Model file for the job. Use its own axes, mm. Face numbers are marked on the shaded views. A direction names the side the tool comes from. Round coordinates to 2 decimals unless told otherwise and drop trailing zeros. Loops run counter-clockwise (first coordinate to the right, second up) from the corner with the lowest first, then second, coordinate; pieces in that order, holes last. Notation, with made-up numbers: M 79.25,59.5 L 126.25,59.5 A29 ccw 126.25,96.5 Z; hole C 79.5,57.5 d1. An arc over 180 degrees is marked long. Answer in a Markdown table with one row per item.
from build123d import *

# Parameters (mm, degrees)
BOSS_EXTRUDE1_DEPTH = 51
CUT_EXTRUDE2_DEPTH  = 51
SKETCH4_R           = 1.625
CUT_EXTRUDE3_DEPTH  = 51
CHAMFER1_SIZE       = 5
FILLET1_R           = 2
SKETCH5_W           = 20.5
SKETCH5_H           = 40.5
CUT_EXTRUDE4_DEPTH  = 10
RIB1_REACH          = 100.443
SKETCH6_WALL_W      = 251.096798658
SKETCH6_WALL_H      = 4
SKETCH7_R           = 1.5
CUT_EXTRUDE5_DEPTH  = 10
SKETCH2_R           = 11.125
CUT_EXTRUDE6_DEPTH  = 10


with BuildPart() as part:
    # Sketch1 → Boss-Extrude1 (new body)
    with BuildSketch(Plane(origin=(0, 0, 0), x_dir=(0, 0, -1), z_dir=(1, 0, 0))):
        Polygon((0, 0), (0, 67), (4, 67), (4, 4), (51, 4), (51, 0), align=None)
    extrude(amount=BOSS_EXTRUDE1_DEPTH)

    # Sketch3 → Cut-Extrude2 (cut)
    with BuildSketch(Plane(origin=(0, 4, 0), x_dir=(1, 0, 0), z_dir=(0, 1, 0))):
        with BuildLine():
            Line((8.34, 40.85), (8.34, 11.15))
            ThreePointArc((8.34, 11.15), (10.49, 9), (12.64, 11.15))
            Line((12.64, 11.15), (12.64, 40.85))
            ThreePointArc((12.64, 40.85), (10.49, 43), (8.34, 40.85))
        make_face()
        with BuildLine():
            Line((38.36, 40.85), (38.36, 11.15))
            ThreePointArc((38.36, 11.15), (40.51, 9), (42.66, 11.15))
            Line((42.66, 11.15), (42.66, 40.85))
            ThreePointArc((42.66, 40.85), (40.51, 43), (38.36, 40.85))
        make_face()
    extrude(amount=-CUT_EXTRUDE2_DEPTH, mode=Mode.SUBTRACT)

    # Sketch4 → Cut-Extrude3 (cut)
    with BuildSketch(Plane.XY):
        with Locations((10, 46.5)):
            Circle(SKETCH4_R)
        with Locations((41, 46.5)):
            Circle(SKETCH4_R)
        with Locations((41, 15.5)):
            Circle(SKETCH4_R)
        with Locations((10, 15.5)):
            Circle(SKETCH4_R)
    extrude(amount=-CUT_EXTRUDE3_DEPTH, mode=Mode.SUBTRACT)

    # Chamfer1
    chamfer1_edges = [part.edges().sort_by_distance(p)[0] for p in [
        (51, 67, -2),
        (0, 67, -2),
        (0, 2, -51),
        (51, 2, -51),
    ]]
    chamfer(chamfer1_edges, length=CHAMFER1_SIZE)

    # Fillet1
    fillet1_edges = [part.edges().sort_by_distance(p)[0] for p in [
        (46, 2, -51),
        (5, 2, -51),
        (0, 62, -2),
        (0, 2, -46),
        (51, 62, -2),
        (51, 2, -46),
        (5, 67, -2),
        (46, 67, -2),
    ]]
    fillet(fillet1_edges, radius=FILLET1_R)

    # Sketch5 → Cut-Extrude4 (cut)
    with BuildSketch(Plane(origin=(0, 0, -4), x_dir=(-1, 0, 0), z_dir=(0, 0, -1))):
        with Locations((-25.5, 36.25)):
            Rectangle(SKETCH5_W, SKETCH5_H)
    extrude(amount=-CUT_EXTRUDE4_DEPTH, mode=Mode.SUBTRACT)

    # Sketch6 wall → Rib1 (add, up to next)
    with BuildSketch(Plane(origin=(51, 21.375514331, -23.483064602), x_dir=(0, -0.665587686923, -0.746319657397), z_dir=(0, 0.746319657397, -0.665587686923)), mode=Mode.PRIVATE) as rib1_sk1:
        with Locations((0, 2)):
            Rectangle(SKETCH6_WALL_W, SKETCH6_WALL_H)
    rib1_tool1 = extrude(rib1_sk1.sketch, amount=-RIB1_REACH, mode=Mode.PRIVATE) - part.part
    rib1 = rib1_tool1.solids().sort_by_distance((51, 21.375514331, -23.483064602))[0]
    add(rib1)

    # Mirror1: Rib1 across plane
    add(rib1.mirror(Plane.ZY.offset(-25.5)))

    # Sketch7 → Cut-Extrude5 (cut)
    with BuildSketch(Plane(origin=(0, 0, -4), x_dir=(-1, 0, 0), z_dir=(0, 0, -1))):
        with Locations(Location((-31.45, 60.8, 0), (0, 0, 90))):
            Circle(SKETCH7_R)
        with Locations(Location((-19.55, 60.8, 0), (0, 0, 90))):
            Circle(SKETCH7_R)
        with Locations(Location((-31.45, 11.7, 0), (0, 0, 90))):
            Circle(SKETCH7_R)
        with Locations(Location((-19.55, 11.7, 0), (0, 0, 90))):
            Circle(SKETCH7_R)
    extrude(amount=-CUT_EXTRUDE5_DEPTH, mode=Mode.SUBTRACT)

    # Sketch2 → Cut-Extrude6 (cut)
    with BuildSketch(Plane.XY):
        with Locations((25.5, 31)):
            Circle(SKETCH2_R)
    extrude(amount=-CUT_EXTRUDE6_DEPTH, mode=Mode.SUBTRACT)


solid = part.part
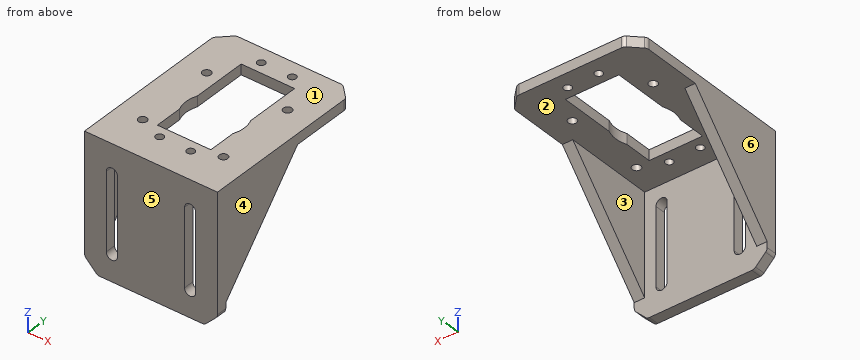
1. Tool access for the marked faces 1 and 2: list every direction of +Z, -Z, +X, -X, +Y, -Y with a clear straight run to the whole face (end or side of a thin tool).
Verdict:
| item | result |
|---|---|
| face 1 | +Z, +X, -X, +Y, -Y |
| face 2 | -Z, +Y |
2. Saw through at C-C (y = 20). Write the cut outline in (x, z).
Verdict:
| item | result |
|---|---|
| outline | M 0,-25.03 L 4,-25.03 L 4,-4 L 15.25,-4 L 15.25,0 L 0,0 Z; M 35.75,-4 L 47,-4 L 47,-25.03 L 51,-25.03 L 51,0 L 35.75,0 Z |
3. Saw through at B-B (z = -26). Write the cut outline in (x, y), and give its area (3 significant figures).
Verdict:
| item | result |
|---|---|
| outline | M 0,0 L 8.34,0 L 8.34,4 L 4,4 L 4,19.13 L 0,19.13 Z; M 12.64,0 L 38.36,0 L 38.36,4 L 12.64,4 Z; M 42.66,0 L 51,0 L 51,19.13 L 47,19.13 L 47,4 L 42.66,4 Z |
| area | 291 mm² |
4. Mould opens along X. For the marked faces 3, 4, 5 and 6 say: +X half, -X half, draft (parallel to the pull), parting line (faces both ways), or undercut.
Verdict:
| item | result |
|---|---|
| face 3 | undercut |
| face 4 | +X half |
| face 5 | draft |
| face 6 | -X half |
5. Pin check, flat tips, straight feed: pin 1 (3 mm diameter, centred on x = 10, y = 46.5, fed in from +Z); pin 2 (14 mm diameter, centred on x = 24, z = -21, fed in from +Y); pin 3 (4 mm diameter, centred on x = 41, y = 46.5, fed in from -Z). Stop position of each tip, or through.
Verdict:
| item | result |
|---|---|
| pin 1 | passes through |
| pin 2 | stops at y = 4 |
| pin 3 | stops at z = -4 |
6. Saw through at A-A (x = 19.55). Write the cut outline in (y, z), and give its area (3 significant figures).
Verdict:
| item | result |
|---|---|
| outline | M 0,-51 L 4,-51 L 4,-4 L 10.2,-4 L 10.2,0 L 0,0 Z; M 13.2,-4 L 16,-4 L 16,0 L 13.2,0 Z; M 56.5,-4 L 59.3,-4 L 59.3,0 L 56.5,0 Z; M 62.3,-4 L 67,-4 L 67,0 L 62.3,0 Z |
| area | 270 mm² |
7. Wall check: probe 1 along X at (y, z) = (60.8, -1.3); probe 2 along Y at (x, z) = (19, -2); probe 3 along Y at (x, z) = (10, -0.9) (3 decimals). Give the ranges that are in metal, low to high.
Verdict:
| item | result |
|---|---|
| probe 1 | x = 0 to 18.05, 21.05 to 29.95, 32.95 to 51 |
| probe 2 | y = 0 to 10.3, 13.1 to 16, 56.5 to 59.4, 62.2 to 67 |
| probe 3 | y = 0 to 13.875, 17.125 to 44.875, 48.125 to 67 |
8. Saw through at D-D (x = 40.51). Write the cut outline in (y, z), and give its area (3 significant figures).
Verdict:
| item | result |
|---|---|
| outline | M 0,-51 L 4,-51 L 4,-43 L 0,-43 Z; M 0,-9 L 4,-9 L 4,-4 L 13.95,-4 L 13.95,0 L 0,0 Z; M 17.05,-4 L 44.95,-4 L 44.95,0 L 17.05,0 Z; M 48.05,-4 L 67,-4 L 67,0 L 48.05,0 Z |
| area | 295 mm² |
